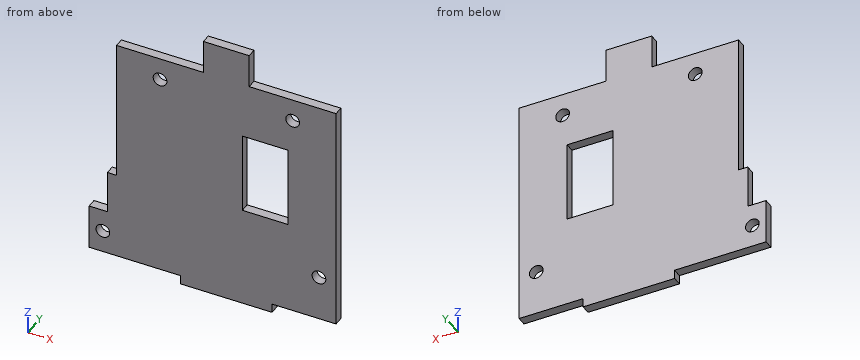
Autodesk Inventor part; units mm, degrees
ref_plane "YZ Plane" through (0, 0, 0) normal (1, 0, 0) x (0, 1, 0)
ref_plane "XZ Plane" through (0, 0, 0) normal (0, 1, 0) x (-1, 0, 0)
ref_plane "XY Plane" through (0, 0, 0) normal (0, 0, 1) x (1, 0, 0)
sketch "Boceto1" plane through (0, 0, 0) normal (0, 1, 0) x (-1, 0, 0)
  line L0 (48, 0) -> (48, -51)
  line L1 (48, -51) -> (0, -51)
  line L2 (0, -51) -> (0, 0)
  line L3 (24, 7.5) -> (29, 7.5)
  line L4 (29, 7.5) -> (29, 0)
  line L5 (24, 7.5) -> (19, 7.5)
  line L6 (19, 7.5) -> (19, 0)
  line L7 (24, 7.5) -> (24, -1.25)
  circle A0 centre (24, -1.25) radius 1.5
  line L8 (29, 0) -> (48, 0)
  line L9 (19, 0) -> (0, 0)
  dimension "d0" = 48
  dimension "d1" = 51
  dimension "d3" = 5
  dimension "d4" = 5
  dimension "d5" = 8.75
  dimension "d6" = 3
extrude "Extrusión1" add sketch "Boceto1" along normal blind 2
ref_plane "Plano de trabajo1" through (-48, -25, -47.5) normal (0, -1, 0) x (1, 0, 0)
sketch "Boceto4" plane through (0, 2, 0) normal (0, 1, 0) x (1, 0, 0)
  line L0 (0, 51) -> (-48, 51)
  line L1 (-24, 51) -> (-24, 53)
  line L2 (-24, 53) -> (-34, 53)
  line L3 (-34, 53) -> (-34, 51)
  line L4 (-34, 51) -> (-14, 51)
  line L5 (-14, 51) -> (-14, 53)
  line L6 (-14, 53) -> (-24, 53)
  point P0 (0, 0)
  dimension "d18" = 2
  dimension "d19" = 10
  dimension "d20" = 20
extrude "Extrusión4" add sketch "Boceto4" against normal blind 2
sketch "Boceto6" plane through (0, 2, 0) normal (0, 1, 0) x (1, 0, 0)
  line L0 (-48, 47.5) -> (-48, 31.5)
  line L1 (-48, 47.5) -> (-18.5, 47.5)
  line L2 (-18.5, 47.5) -> (-18.5, 26.5)
  line L3 (-18.5, 26.5) -> (-18.5, 16.5)
  line L4 (-18.5, 16.5) -> (-12.5, 16.5)
  line L5 (-12.5, 16.5) -> (-12.5, 26.5)
  line L6 (-12.5, 26.5) -> (-18.5, 26.5)
  point P0 (0, 0)
  dimension "d26" = 29.5
  dimension "d27" = 21
  dimension "d28" = 10
  dimension "d29" = 6
extrude "Extrusión6" cut sketch "Boceto6" against normal blind 2
sketch "Boceto7" plane through (0, 2, 0) normal (0, 1, 0) x (1, 0, 0)
  circle A0 centre (-24, 1.25) radius 1.5
  circle A1 centre (-24, 1.25) radius 1.5
  point P0 (0, 0)
extrude "Extrusión7" add sketch "Boceto7" against normal blind 2
sketch "Boceto8" plane through (0, 2, 0) normal (0, 1, 0) x (1, 0, 0)
  line L0 (-48, 51) -> (-48, 0)
  line L1 (-48, 51) -> (-48, 31.5)
  line L2 (-48, 31.5) -> (-50, 31.5)
  line L3 (-50, 31.5) -> (-50, 41)
  line L4 (-50, 41) -> (-54, 41)
  line L5 (-54, 41) -> (-54, 51)
  line L6 (-54, 51) -> (-48, 51)
  point P0 (0, 0)
  dimension "d34" = 19.5
  dimension "d35" = 2
  dimension "d36" = 9.5
  dimension "d37" = 4
extrude "Extrusión8" add sketch "Boceto8" against normal blind 2
sketch "Boceto9" plane through (0, 2, 0) normal (0, 1, 0) x (1, 0, 0)
  line L0 (-48, 0) -> (-29, 0)
  line L1 (-48, 0) -> (-48, 5)
  line L2 (-48, 31.5) -> (-48, 0)
  line L3 (-48, 5) -> (-38.5, 5)
  line L4 (-48, 5) -> (-9.5, 5)
  circle A0 centre (-38.5, 5) radius 1.5
  circle A1 centre (-9.5, 5) radius 1.5
  line L5 (0, 51) -> (-14, 51)
  line L6 (0, 51) -> (0, 41)
  line L7 (0, 0) -> (0, 51)
  line L8 (0, 41) -> (-3.75, 41)
  circle A2 centre (-3.75, 41) radius 1.5
  line L9 (-34, 51) -> (-54, 51)
  line L10 (-54, 51) -> (-51, 51)
  line L11 (-51, 51) -> (-51, 46)
  circle A3 centre (-51, 46) radius 1.5
  dimension "d40" = 5
  dimension "d41" = 9.5
  dimension "d42" = 38.5
  dimension "d43" = 3
  dimension "d44" = 3
  dimension "d45" = 10
  dimension "d46" = 3.75
  dimension "d47" = 3
  dimension "d48" = 3
  dimension "d49" = 3
extrude "Extrusión9" cut sketch "Boceto9" against normal blind 2
sketch "Boceto10" plane through (0, 2, 0) normal (0, 1, 0) x (1, 0, 0)
  line L0 (-18.5, 16.5) -> (-18.5, 26.5)
  line L1 (-20.5, 16.5) -> (-20.5, 12.5)
  line L2 (-20.5, 12.5) -> (-12.5, 12.5)
  line L3 (-12.5, 12.5) -> (-10.5, 12.5)
  line L4 (-10.5, 12.5) -> (-10.5, 26.5)
  line L5 (-10.5, 26.5) -> (-10.5, 30.5)
  line L6 (-10.5, 30.5) -> (-18.5, 30.5)
  line L7 (-18.5, 30.5) -> (-20.5, 30.5)
  line L8 (-20.5, 16.5) -> (-20.5, 30.5)
  point P0 (0, 0)
  dimension "d52" = 2
  dimension "d53" = 4
  dimension "d54" = 2
  dimension "d55" = 4
extrude "Extrusión10" cut sketch "Boceto10" against normal blind 10
properties part number "arm_2_case"
Check sheet for the modelled part. Datum: model origin and axes. Units: mm. Round coordinates to 2 decimals unless told otherwise and drop trailing zeros. Order: outer loops, then holes, each group sorted by start corner. A loop starts at its lowest first (then second) coordinate and runs counter-clockwise, first axis right, second up.
(1) Scan lines: probe 1 along X at (y, z) = (0.75, -5); probe 2 along Z at (x, y) = (-38.5, 0.7); probe 3 along X at (y, z) = (1.85, -23.5). Record each from-to range of solid material in increasing order.
(2) Cross-section at D-D, the plane z = -5. Enter the section's corners in (x, y).
(3) Cross-section at B-B, the plane z = -14. Enter the section's corners in (x, y), and give its area (3 significant figures).
(4) Cross-section at C-C, the plane y = 1.25. Enter the section's corners in (x, z).
(5) Go/stop test with flat-tipped pins: P1, Ø0.6, axis at x = -16, y = 1.5, coming from the +Z side; P2, Ø0.6, axis at y = 0.5, z = 5.5, coming from the -X side; P3, Ø1, axis at y = 0.5, z = -34.5, coming from the -X side. Record where each tip stops, or that it passes through.
(6) Cross-section at A-A, the plane x = -12.5. Enter the section's corners in (y, z), and give its area (3 significant figures).
Check sheet entries:
1. probe 1: x = -48 to -40, -37 to -11, -8 to 0
1. probe 2: z = -51 to -6.5, -3.5 to 0
1. probe 3: x = -48 to -20.5, -10.5 to 0
2. outline: (-48, 0) - (-40, 0) - (-40, 2) - (-48, 2) - close; (-37, 0) - (-11, 0) - (-11, 2) - (-37, 2) - close; (-8, 0) - (0, 0) - (0, 2) - (-8, 2) - close
3. outline: (-48, 0) - (-20.5, 0) - (-20.5, 2) - (-48, 2) - close; (-10.5, 0) - (0, 0) - (0, 2) - (-10.5, 2) - close
3. area: 76.0 mm2
4. outline: (-54, -51) - (-34, -51) - (-34, -53) - (-14, -53) - (-14, -51) - (0, -51) - (0, 0) - (-19, 0) - (-19, 7.5) - (-29, 7.5) - (-29, 0) - (-48, 0) - (-48, -31.5) - (-50, -31.5) - (-50, -41) - (-54, -41) - close; hole circle Ø3 at (-51, -46); hole circle Ø3 at (-38.5, -5); hole (-20.5, -30.5) - (-10.5, -30.5) - (-10.5, -12.5) - (-20.5, -12.5) - close; hole circle Ø3 at (-9.5, -5); hole circle Ø3 at (-3.75, -41)
5. P1: stops at z = 0
5. P2: stops at x = -29
5. P3: stops at x = -50
6. outline: (0, -51) - (2, -51) - (2, -30.5) - (0, -30.5) - close; (0, -12.5) - (2, -12.5) - (2, 0) - (0, 0) - close
6. area: 66.0 mm2
